Read the model definition and answer for the solid it produces. Units are mm, in the model's axes. Coordinates: 2 decimals unless noted, no trailing zeros. Write each loop counter-clockwise with the first axis right and the second up, starting at its lowest first coordinate (ties: lowest second). Pieces come first, ordered by that corner, then holes.
Item 1: Section C-C (z = 0.45) is taken. State how many separate pieces and enclosed holes the cut face has, then the cut area to 3 significant figures.
Item 2: Determine the mould class of faces 1 (the face through (33.73, -45.42, 0.79)), 2 (the face through (-1, 1, 1.6)), 3 (the face through (38.313, 47.762, 0.789)) for opening direction X: released by +X, released by -X, zero draft, split by the parting line, or undercut.
Item 3: Straight lines are drawn through the part: probe 1 along Y at (x, z) = (-6.29, 1.2); probe 2 along X at (y, z) = (4, 0.4) (3 decimals); probe 3 along Y at (x, z) = (-25, 0.8). For each, find the intervals that lie inside material, in ascending order.
Item 4: Section A-A (x = -25) is taken. Give the vertices of the cut face in (y, z), then the cut area to 3 significant figures.
Item 5: Section B-B (y = -9.2) is taken. Give the vertices of the cut face in (x, z) (3 decimals), then the cut area to 3 significant figures.
Autodesk Inventor part; units mm, degrees
ref_plane "YZ Plane" through (0, 0, 0) normal (1, 0, 0) x (0, 1, 0)
ref_plane "XZ Plane" through (0, 0, 0) normal (0, 1, 0) x (-1, 0, 0)
ref_plane "XY Plane" through (0, 0, 0) normal (0, 0, 1) x (1, 0, 0)
sketch "Sketch1" plane through (0, 0, 0) normal (0, 0, 1) x (1, 0, 0)
  line L0 (-41.275, -50.8) -> (41.275, -50.8)
  line L1 (41.275, -50.8) -> (41.275, 50.8)
  line L2 (41.275, 50.8) -> (-41.275, 50.8)
  line L3 (-41.275, 50.8) -> (-41.275, -50.8)
  line L4 (-41.275, -50.8) -> (41.275, 50.8) construction
  line L5 (41.275, -50.8) -> (-41.275, 50.8) construction
  circle A0 centre (-35, -46.39) radius 1.6
  circle A1 centre (35, -46.39) radius 1.6
  point P0 (0, 0)
  dimension "d0" = 82.55
  dimension "d1" = 101.6
  dimension "d2" = 3.2
  dimension "d3" = 3.2
  dimension "d5" = 35
  dimension "d6" = 35
  dimension "d7" = 4.41
  dimension "d8" = 4.41
extrude "Extrusion1" add sketch "Sketch1" along normal blind 1.6
chamfer "Chamfer1" distance 6 angle 45 1 edges at (41.275, 50.8, 0.8) measured on face at (41.275, -16.9333, 0.5333)
chamfer "Chamfer2" distance 6 angle 45 1 edges at (-41.275, 50.8, 0.8) measured on face at (-41.275, 16.9333, 0.5333)
sketch "Sketch2" plane through (0, 0, 1.6) normal (0, 0, 1) x (1, 0, 0)
  circle A0 centre (-10.48, -42) radius 0.52
  line L0 (-41.275, -50.8) -> (41.275, -50.8)
  line L1 (-41.275, 44.8) -> (-41.275, -50.8)
  point P0 (0, 0)
  dimension "d17" = 1.04
  dimension "d18" = 10.48
  dimension "d19" = 8.8
extrude "Extrusion2" cut sketch "Sketch2" against normal through all
pattern_linear "Rectangular Pattern1" count 6 spacing 4.19 along (1, 0, 0) count 2 spacing 6.35 along (0, -1, 0) of "Extrusion2"
sketch "Sketch3" plane through (0, 0, 1.6) normal (0, 0, 1) x (1, 0, 0)
  circle A0 centre (-25, 20.8) radius 1.6
  circle A1 centre (-25, -9.2) radius 1.6
  line L0 (0, -71.12) -> (0, 71.12)
  line L1 (35.275, 50.8) -> (-35.275, 50.8)
  circle A2 centre (25, 20.8) radius 1.6
  circle A3 centre (25, -9.2) radius 1.6
  point P0 (0, 0)
  dimension "d28" = 25
  dimension "d29" = 25
  dimension "d30" = 30
  dimension "d31" = 3.2
  dimension "d32" = 3.2
  dimension "d33" = 30
extrude "Extrusion3" cut sketch "Sketch3" against normal through all
sketch "Sketch4" plane through (0, 0, 1.6) normal (0, 0, 1) x (1, 0, 0)
  line L0 (-16, 0) -> (-16, 4) construction
  line L1 (-14.5, 0) -> (-14.5, 4)
  line L2 (-17.5, 4) -> (-17.5, 0)
  arc A0 (-17.5, 0) -> (-14.5, 0) centre (-16, 0) ccw
  arc A1 (-14.5, 4) -> (-17.5, 4) centre (-16, 4) ccw
  line L3 (-16, 25) -> (-16, 29) construction
  line L4 (-14.5, 25) -> (-14.5, 29)
  line L5 (-17.5, 29) -> (-17.5, 25)
  arc A2 (-17.5, 25) -> (-14.5, 25) centre (-16, 25) ccw
  arc A3 (-14.5, 29) -> (-17.5, 29) centre (-16, 29) ccw
  line L6 (-57.785, 0) -> (57.785, 0) construction
  line L7 (0, 71.12) -> (0, -71.12)
  line L8 (16, 0) -> (16, 4) construction
  line L9 (14.5, 0) -> (14.5, 4)
  line L10 (17.5, 4) -> (17.5, 0)
  arc A4 (14.5, 0) -> (17.5, 0) centre (16, 0) ccw
  arc A5 (17.5, 4) -> (14.5, 4) centre (16, 4) ccw
  line L11 (16, 25) -> (16, 29) construction
  line L12 (14.5, 25) -> (14.5, 29)
  line L13 (17.5, 29) -> (17.5, 25)
  arc A6 (14.5, 25) -> (17.5, 25) centre (16, 25) ccw
  arc A7 (17.5, 29) -> (14.5, 29) centre (16, 29) ccw
  line L14 (13.3, -8.625) -> (-13.3, -8.625)
  line L15 (-13.3, -8.625) -> (-13.3, 37.625)
  line L16 (-13.3, 37.625) -> (13.3, 37.625)
  line L17 (13.3, 37.625) -> (13.3, -8.625)
  line L18 (13.3, -8.625) -> (-13.3, 37.625) construction
  line L19 (-13.3, -8.625) -> (13.3, 37.625) construction
  point P0 (0, 0)
  point P1 (-16, 2)
  point P2 (-16, 27)
  point P3 (16, 2)
  point P4 (16, 27)
  point P5 (0, 14.5)
  dimension "d36" = 4
  dimension "d37" = 4
  dimension "d38" = 3
  dimension "d39" = 3
  dimension "d40" = 16
  dimension "d41" = 25
  dimension "d45" = 26.6
  dimension "d46" = 46.25
  dimension "d47" = 12.5
  dimension "d48" = 2
extrude "Extrusion4" cut sketch "Sketch4" against normal blind 1.6 contours A0 L2 A1 L1 | A2 L5 A3 L4 | L9 A5 L10 A4 | L12 A7 L13 A6
fillet "Fillet1" radius 1 6 edges at (41.275, -50.8, 0.8) (41.275, 44.8, 0.8) (35.275, 50.8, 0.8) (-35.275, 50.8, 0.8) (-41.275, 44.8, 0.8) (-41.275, -50.8, 0.8)
sketch "RCU_PCB_OUTLINE" plane through (0, 0, 1.6) normal (0, 0, 1) x (1, 0, 0)
  circle A0 centre (-25, 20.8) radius 1.6
  circle A1 centre (25, 20.8) radius 1.6
  circle A2 centre (-25, -9.2) radius 1.6
  circle A3 centre (25, -9.2) radius 1.6
  circle A4 centre (10.47, -48.35) radius 0.52
  circle A5 centre (-10.48, -42) radius 0.52
  circle A6 centre (-35, -46.39) radius 1.6
  circle A7 centre (35, -46.39) radius 1.6
  line L0 (-30, -13.2) -> (-30, 24.8)
  line L1 (-30, -13.2) -> (-30, 24.8)
  arc A8 (-30, -13.2) -> (-29, -14.2) centre (-29, -13.2) ccw
  arc A9 (-29, 25.8) -> (-30, 24.8) centre (-29, 24.8) ccw
  arc A10 (-30, -13.2) -> (-29, -14.2) centre (-29, -13.2) ccw
  line L2 (-21, -14.2) -> (-29, -14.2)
  arc A11 (-21, -14.2) -> (-20, -13.2) centre (-21, -13.2) ccw
  line L3 (-20, 24.8) -> (-20, -13.2)
  arc A12 (-20, 24.8) -> (-21, 25.8) centre (-21, 24.8) ccw
  line L4 (-29, 25.8) -> (-21, 25.8)
  arc A13 (-29, 25.8) -> (-30, 24.8) centre (-29, 24.8) ccw
  arc A14 (12.3, -8.625) -> (13.3, -7.625) centre (12.3, -7.625) ccw
  line L5 (-12.3, -8.625) -> (12.3, -8.625)
  arc A15 (-13.3, -7.625) -> (-12.3, -8.625) centre (-12.3, -7.625) ccw
  line L6 (-13.3, 36.625) -> (-13.3, -7.625)
  arc A16 (-12.3, 37.625) -> (-13.3, 36.625) centre (-12.3, 36.625) ccw
  line L7 (12.3, 37.625) -> (-12.3, 37.625)
  arc A17 (13.3, 36.625) -> (12.3, 37.625) centre (12.3, 36.625) ccw
  line L8 (13.3, -7.625) -> (13.3, 36.625)
  line L9 (29, -14.2) -> (21, -14.2)
  arc A18 (20, -13.2) -> (21, -14.2) centre (21, -13.2) ccw
  line L10 (20, -13.2) -> (20, 24.8)
  arc A19 (21, 25.8) -> (20, 24.8) centre (21, 24.8) ccw
  line L11 (21, 25.8) -> (29, 25.8)
  arc A20 (30, 24.8) -> (29, 25.8) centre (29, 24.8) ccw
  line L12 (30, 24.8) -> (30, -13.2)
  arc A21 (29, -14.2) -> (30, -13.2) centre (29, -13.2) ccw
  line L13 (29, -14.2) -> (21, -14.2)
  arc A22 (14.5, 0) -> (17.5, 0) centre (16, 0) ccw
  line L14 (17.5, 4) -> (17.5, 0)
  arc A23 (17.5, 4) -> (14.5, 4) centre (16, 4) ccw
  line L15 (14.5, 0) -> (14.5, 4)
  arc A24 (-17.5, 0) -> (-14.5, 0) centre (-16, 0) ccw
  line L16 (-14.5, 4) -> (-14.5, 0)
  arc A25 (-14.5, 4) -> (-17.5, 4) centre (-16, 4) ccw
  line L17 (-17.5, 0) -> (-17.5, 4)
  arc A26 (-17.5, 25) -> (-14.5, 25) centre (-16, 25) ccw
  line L18 (-14.5, 29) -> (-14.5, 25)
  arc A27 (-14.5, 29) -> (-17.5, 29) centre (-16, 29) ccw
  line L19 (-17.5, 25) -> (-17.5, 29)
  arc A28 (14.5, 25) -> (17.5, 25) centre (16, 25) ccw
  line L20 (17.5, 29) -> (17.5, 25)
  arc A29 (17.5, 29) -> (14.5, 29) centre (16, 29) ccw
  line L21 (14.5, 25) -> (14.5, 29)
  line L22 (41.275, -49.8) -> (41.275, 44.3858)
  arc A30 (40.275, -50.8) -> (41.275, -49.8) centre (40.275, -49.8) ccw
  line L23 (-40.275, -50.8) -> (40.275, -50.8)
  arc A31 (-41.275, -49.8) -> (-40.275, -50.8) centre (-40.275, -49.8) ccw
  line L24 (-41.275, 44.3858) -> (-41.275, -49.8)
  arc A32 (-40.9821, 45.0929) -> (-41.275, 44.3858) centre (-40.275, 44.3858) ccw
  line L25 (-40.9821, 45.0929) -> (-35.5679, 50.5071)
  arc A33 (-34.8608, 50.8) -> (-35.5679, 50.5071) centre (-34.8608, 49.8) ccw
  line L26 (34.8608, 50.8) -> (-34.8608, 50.8)
  arc A34 (35.5679, 50.5071) -> (34.8608, 50.8) centre (34.8608, 49.8) ccw
  line L27 (35.5679, 50.5071) -> (40.9821, 45.0929)
  arc A35 (41.275, 44.3858) -> (40.9821, 45.0929) centre (40.275, 44.3858) ccw
  point P0 (0, 0)
equation "\"d8\" = d7"
equation "\"d32\" = d31"
equation "\"d37\" = d36"
equation "\"d39\" = d38"
properties part number "PCB"
Established:
1. separate pieces: 1
1. enclosed holes: 22
1. area: 8,220 mm2
2. face 1: undercut
2. face 2: zero draft
2. face 3: released by +X
3. probe 1: y = -50.8 to -48.87, -47.83 to -42.52, -41.48 to 50.8
3. probe 2: x = -41.275 to -17.5, -14.5 to 14.5, 17.5 to 41.275
3. probe 3: y = -50.8 to -10.8, -7.6 to 19.2, 22.4 to 50.8
4. outline: (-50.8, 0) - (-10.8, 0) - (-10.8, 1.6) - (-50.8, 1.6) - close; (-7.6, 0) - (19.2, 0) - (19.2, 1.6) - (-7.6, 1.6) - close; (22.4, 0) - (50.8, 0) - (50.8, 1.6) - (22.4, 1.6) - close
4. area: 152 mm2
5. outline: (-41.275, 0) - (-26.6, 0) - (-26.6, 1.6) - (-41.275, 1.6) - close; (-23.4, 0) - (23.4, 0) - (23.4, 1.6) - (-23.4, 1.6) - close; (26.6, 0) - (41.275, 0) - (41.275, 1.6) - (26.6, 1.6) - close
5. area: 122 mm2
